Job drawing, mm, ordinate dimensions from the low corner. One solid piece. Coordinates: 2 decimals unless noted, no trailing zeros. Write each loop counter-clockwise with the first axis right and the second up, starting at its lowest first coordinate (ties: lowest second). Pieces come first, ordered by that corner, then holes. Notation, with made-up numbers: (67, 12) - (98, 12) arc R24 ccw to (98, 39) - close; hole circle Ø3 at (80, 3). An arc over 180 degrees is marked (long way). Use one line per item in the form item = value. Start each with the question number.
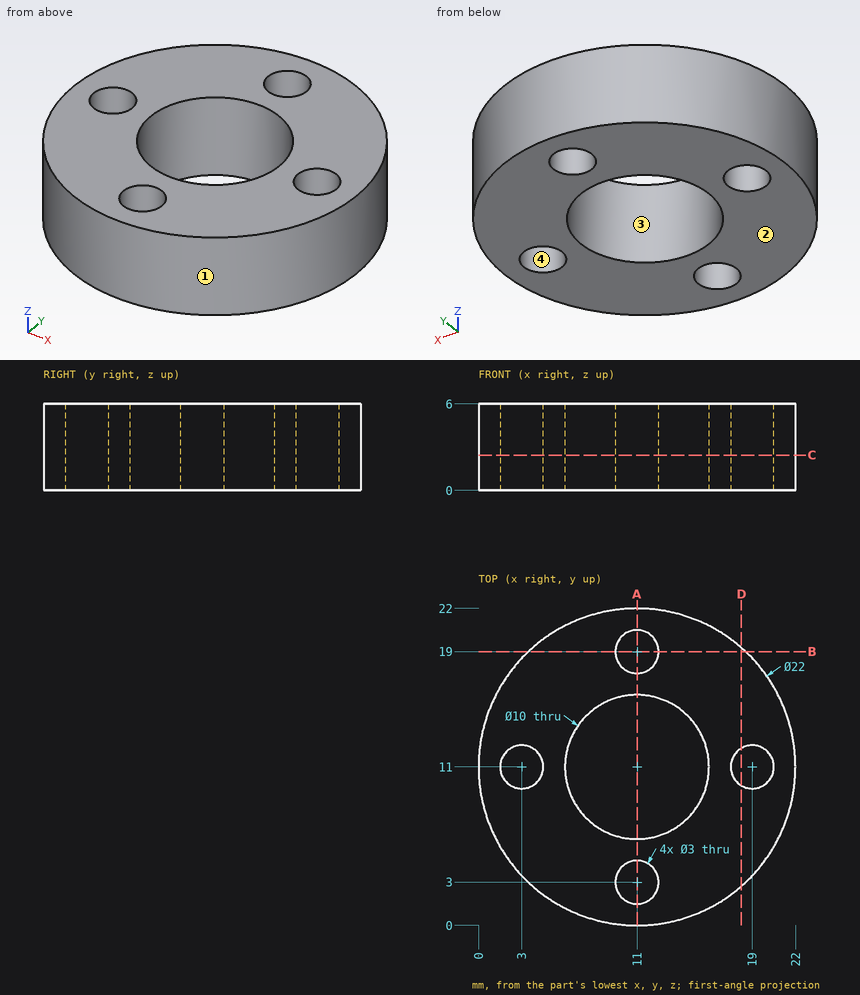
Q1. Pin check, flat tips, straight feed: P1, Ø1, axis at y = 6, z = 2.5, coming from the +X side; P2, Ø1.5, axis at y = 7.5, z = 2.5, coming from the +X side; P3, Ø2.5, axis at x = 19, y = 11, coming from the -Z side; P4, Ø2, axis at y = 15.5, z = 4, coming from the -X side. Stop position of each tip, or through.
Q2. Mould opens along X. For the marked faces 1, 2, 3 and 4 say: released by +X, released by -X, zero draft, split by the parting line, or undercut.
Q3. Slice it at D-D (x = 18.25). List the corners of the cut face in (y, z).
Q4. Slice it at A-A (x = 11). List the corners of the cut face in (y, z).
Q5. Slice it at C-C (z = 2.45). List the corners of the cut face in (x, y).
Q6. Slice it at B-B (y = 19). List the corners of the cut face in (x, z), plus the area to 3 significant figures.
Q7. Drill centre lines: probe 1 along Y at (x, z) = (11, 2.65); probe 2 along Y at (x, z) = (10.25, 5.2); probe 3 along X at (y, z) = (14.5, 2.25). Where is each one in solid material? Low to high.
Solution:
q1.P1 = 21.04
q1.P2 = 21.65
q1.P3 = through
q1.P4 = 0.57
q2.face_1 = split by the parting line
q2.face_2 = zero draft
q2.face_3 = undercut
q2.face_4 = undercut
q3.outline = (2.73, 0) - (9.7, 0) - (9.7, 6) - (2.73, 6) - close; (12.3, 0) - (19.27, 0) - (19.27, 6) - (12.3, 6) - close
q4.outline = (0, 0) - (1.5, 0) - (1.5, 6) - (0, 6) - close; (4.5, 0) - (6, 0) - (6, 6) - (4.5, 6) - close; (16, 0) - (17.5, 0) - (17.5, 6) - (16, 6) - close; (20.5, 0) - (22, 0) - (22, 6) - (20.5, 6) - close
q5.outline = circle Ø22 at (11, 11); hole circle Ø3 at (3, 11); hole circle Ø10 at (11, 11); hole circle Ø3 at (11, 3); hole circle Ø3 at (11, 19); hole circle Ø3 at (19, 11)
q6.outline = (3.45, 0) - (9.5, 0) - (9.5, 6) - (3.45, 6) - close; (12.5, 0) - (18.55, 0) - (18.55, 6) - (12.5, 6) - close
q6.area = 72.6 mm2
q7.probe_1 = 0 to 1.5, 4.5 to 6, 16 to 17.5, 20.5 to 22
q7.probe_2 = 0.03 to 1.7, 4.3 to 6.06, 15.94 to 17.7, 20.3 to 21.97
q7.probe_3 = 0.57 to 7.43, 14.57 to 21.43
